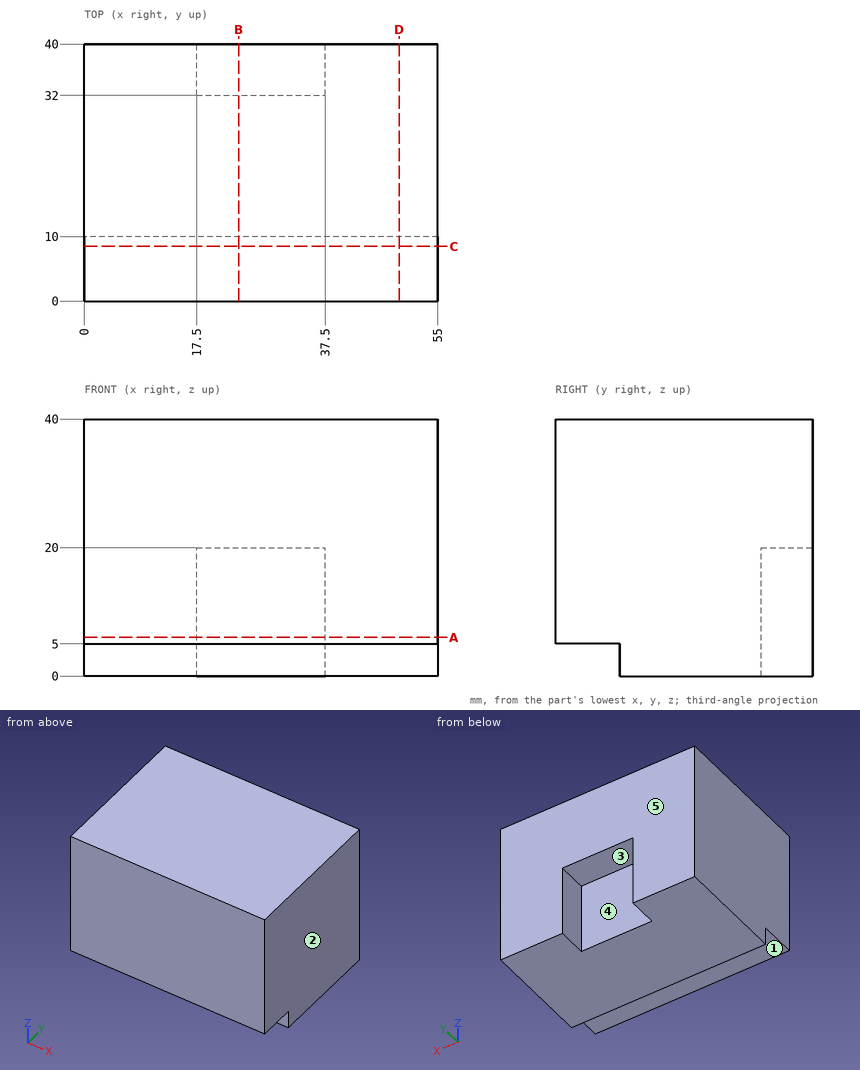
Geometry check sheet. Reference: drawing and pictorial views, mm from the part's lowest x, y, z. A direction names the side the tool comes from. Give positions to 0.01 mm unless a question says otherwise; leave off trailing zeros. Write each loop counter-clockwise with the first axis right and the second up, starting at its lowest first coordinate (ties: lowest second). Pieces come first, ordered by that corner, then holes. Notation, with made-up numbers: (67.5, 37.25) - (78.5, 37.25) arc R30 ccw to (78.5, 74.25) - close; hole circle Ø5 at (82.5, 56). An arc over 180 degrees is marked (long way). Use a Markdown table: item, result.
Q1. Section check C-C, the plane y = 8.5. Enter the section's corners in (x, z), then the cut area to 4 significant figures.
Computed:
| item | result |
|---|---|
| outline | (0, 5) - (55, 5) - (55, 40) - (0, 40) - close |
| area | 1,925 mm² |
Q2. Go/stop test with a flat-tipped pin: P1, Ø10, axis at x = 30.5, z = 8.5, coming from the +Y side. Record where the tip stops, or that it passes through.
Computed:
| item | result |
|---|---|
| P1 | stops at y = 32 |
Q3. Set-up check for the marked faces 4 and 5: record each of +Z, -Z, +X, -X, +Y, -Y from which the full face is reachable in a straight line by a thin tool's end or side.
Computed:
| item | result |
|---|---|
| face 4 | -Z, +Y |
| face 5 | +Z, -Z, +X, -X, +Y |
Q4. Section check D-D, the plane x = 49. Enter the section's corners in (y, z), then the cut area to 3 significant figures.
Computed:
| item | result |
|---|---|
| outline | (0, 5) - (10, 5) - (10, 0) - (40, 0) - (40, 40) - (0, 40) - close |
| area | 1,550 mm² |
Q5. Thickness scan on L1, parallel to Y at x = 22, z = 19; L2, parallel to Z at x = 26, y = 34.5; L3, parallel to Z at x = 28.5, y = 5. Record the ranges inside material, lowest first. Write a range as [from, to].
Computed:
| item | result |
|---|---|
| L1 | y = [0, 32] |
| L2 | z = [20, 40] |
| L3 | z = [5, 40] |
Q6. Section check A-A, the plane z = 6. Enter the section's corners in (x, y), then the cut area to 3 significant figures.
Computed:
| item | result |
|---|---|
| outline | (0, 0) - (55, 0) - (55, 40) - (37.5, 40) - (37.5, 32) - (17.5, 32) - (17.5, 40) - (0, 40) - close |
| area | 2,040 mm² |
Q7. Draft check along X on the marked faces 1, 2 and 3. Enter one of: pulls with the +X half, pulls with the -X half, needs draft (parallel to the pull), parting line crosses it, or undercut.
Computed:
| item | result |
|---|---|
| face 1 | needs draft |
| face 2 | pulls with the +X half |
| face 3 | undercut |
Q8. Section check B-B, the plane x = 24. Enter the section's corners in (y, z).
Computed:
| item | result |
|---|---|
| outline | (0, 5) - (10, 5) - (10, 0) - (32, 0) - (32, 20) - (40, 20) - (40, 40) - (0, 40) - close |
